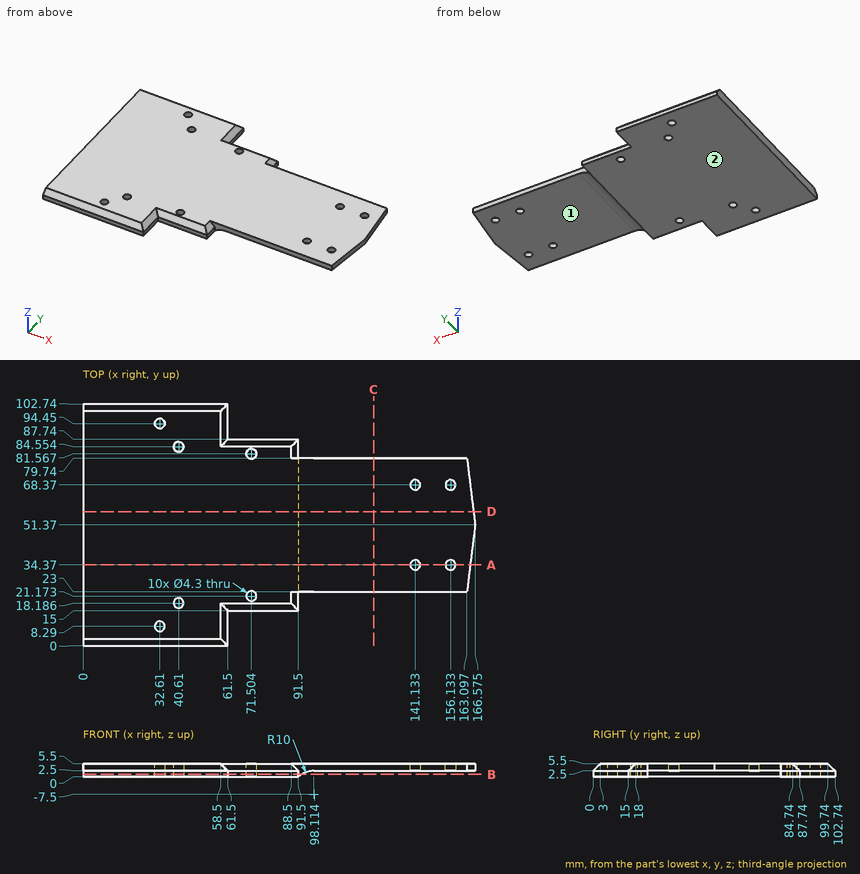
Verification items for this drawing (mm, ordinates from the low corner). A direction names the side the tool comes from. Give positions to 0.01 mm unless a question says otherwise; leave off trailing zeros. Loops run counter-clockwise (first coordinate to the right, second up) from the corner with the lowest first, then second, coordinate; pieces in that order, holes last.
(1) Section check D-D on y = 57. Record the cut outline in (x, z) (1 decimal).
From the geometry:
outline: (0, 0) - (91.5, 0) arc R10 cw to (98.1, 2.5) - (165.9, 2.5) - (165.9, 5.5) - (0, 5.5) - close
(2) Section check B-B on z = 1. Record the cut outline in (x, y), then the cut area to 3 significant figures.
From the geometry:
outline: (0, 0) - (61.5, 0) - (61.5, 15) - (91.5, 15) - (91.5, 23) - (92.85, 23) - (92.85, 79.74) - (91.5, 79.74) - (91.5, 87.74) - (61.5, 87.74) - (61.5, 102.74) - (0, 102.74) - close; hole circle Ø4.3 at (32.61, 8.29); hole circle Ø4.3 at (32.61, 94.45); hole circle Ø4.3 at (40.61, 18.19); hole circle Ø4.3 at (40.61, 84.55); hole circle Ø4.3 at (71.5, 21.17); hole circle Ø4.3 at (71.5, 81.57)
area: 8,490 mm2
(3) Section check A-A on y = 34.37. Record the cut outline in (x, z) (1 decimal).
From the geometry:
outline: (0, 0) - (91.5, 0) arc R10 cw to (98.1, 2.5) - (139, 2.5) - (139, 5.5) - (0, 5.5) - close; (143.3, 2.5) - (154, 2.5) - (154, 5.5) - (143.3, 5.5) - close; (158.3, 2.5) - (164.5, 2.5) - (164.5, 5.5) - (158.3, 5.5) - close
(4) Thickness scan on L1, parallel to X at y = 84.5, z = 0.6; L2, parallel to Z at x = 147, y = 36.5; L3, parallel to Y at x = 101, z = 4.35. Record the ranges inside material, lowest first.
From the geometry:
L1: x = 0 to 38.46, 42.76 to 91.5
L2: z = 2.5 to 5.5
L3: y = 23 to 79.74
(5) Set-up check for the marked faces 1 and 2: record each of +Z, -Z, +X, -X, +Y, -Y from which the full face is reachable in a straight line by a thin tool's end or side.
From the geometry:
face 1: -Z, +X, +Y, -Y
face 2: -Z, +X, -X, +Y, -Y
(6) Depth check by flat-ended pin: pin 1 Ø0.8 at (x, z) = (70.5, 1.5) entering from +Y; pin 2 Ø2 at (x, z) = (77.5, 1) entering from -Y; pin 3 Ø2 at (y, z) = (19.5, 1.5) entering from +X. Enter the tip coordinate at first touch or a pass-through.
From the geometry:
pin 1: stops at y = 87.74
pin 2: stops at y = 15
pin 3: stops at x = 91.5
(7) Section check C-C on x = 123.5. Record the cut outline in (y, z).
From the geometry:
outline: (23, 2.5) - (79.74, 2.5) - (79.74, 5.5) - (23, 5.5) - close
